Input: dimensioned drawing with shaded views. Units: mm. Origin: part minimum x, y, z. A direction names the side the tool comes from. Round coordinates to 2 decimals unless told otherwise and drop trailing zeros. Write each loop counter-clockwise with the first axis right and the second up, starting at its lowest first coordinate (ties: lowest second). Pieces come first, ordered by that corner, then holes. Notation, with made-up numbers: M 60,19.25 L 70,19.25 A26 ccw 70,42.25 Z; hole C -22.75,30 d5. An arc over 180 degrees is marked long. Answer in a Markdown table with one row per item. Add a question column.
Item 1: Cut plane C-C on x = 8.75. Return loops of the section in (y, z).
Item 2: Set-up query: the marked faces 1, 2, 3 and 4. Return all of +Z, -Z, +X, -X, +Y, -Y with unobstructed straight access to the full face (end or side cutting, diameter ignored); none if empty.
Item 3: Cut plane A-A on y = 10. Return loops of the section in (x, z).
Item 4: Contact query for flat-ended pins moving along their axis: pin 1 (3 mm diameter, centred on x = 9, y = 5.5, fed in from +Z); pin 2 (3 mm diameter, centred on x = 9.5, z = 5, fed in from +Y); pin 3 (2 mm diameter, centred on y = 13, z = 8, fed in from +X); pin 4 (3 mm diameter, centred on y = 14, z = 9.5, fed in from -X). Output: stop coordinate, or through.
Item 5: Cut plane B-B on z = 5. Return loops of the section in (x, y).
Item 6: Cut plane D-D on z = 8.5. Return loops of the section in (x, y), and give its area (3 significant figures).
Item 7: Mould query, pull axis Y, two halves, no side actions, for the marked faces 5, 6 and 7. Classes: released by +Y, released by -Y, zero draft, split by the parting line, or undercut.
Item 8: Material intervals for probe 1 along X at (y, z) = (10, 22.35); probe 2 along Z at (x, y) = (9.5, 13.4); probe 3 along X at (y, z) = (10, 18.6), sorted ascending.
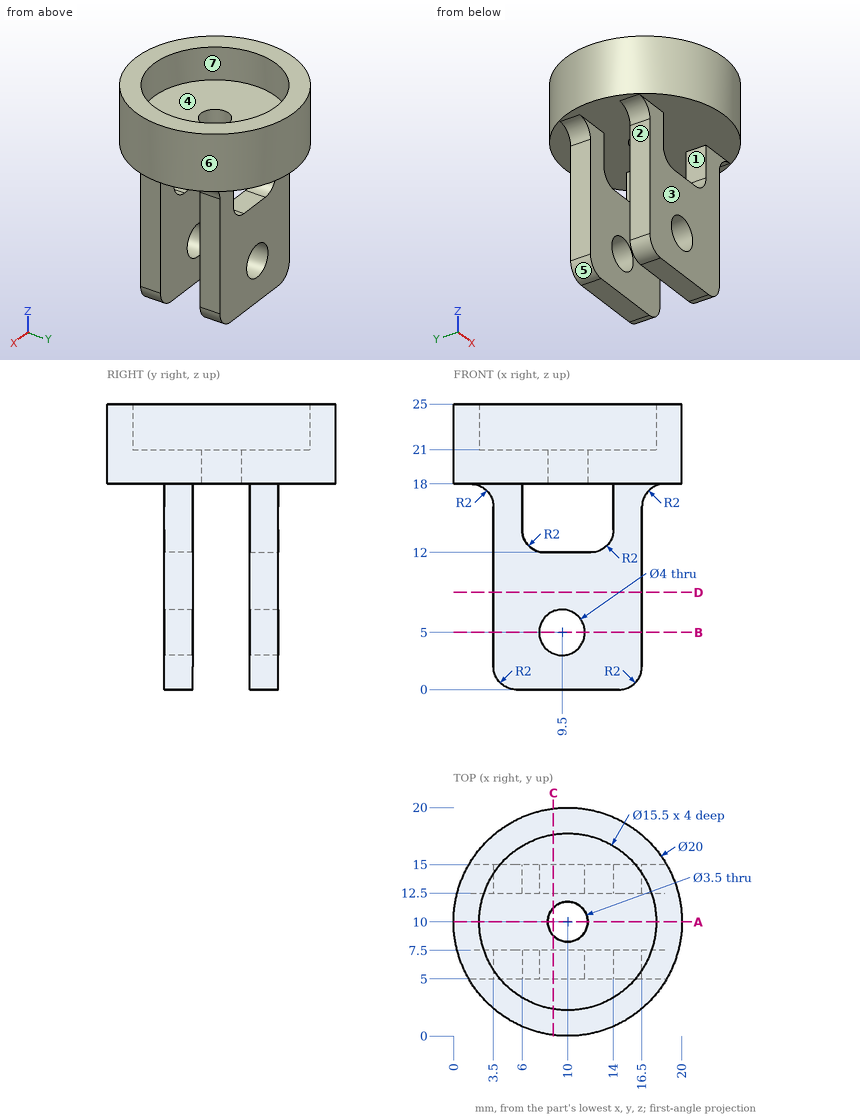
Results below:
| question | item | result |
|---|---|---|
| 1 | outline | M 0.08,18 L 8.78,18 L 8.78,21 L 2.35,21 L 2.35,25 L 0.08,25 Z; M 5,0 L 7.5,0 L 7.5,3.15 L 5,3.15 Z; M 5,6.85 L 7.5,6.85 L 7.5,12 L 5,12 Z; M 11.22,18 L 19.92,18 L 19.92,25 L 17.65,25 L 17.65,21 L 11.22,21 Z; M 12.5,0 L 15,0 L 15,3.15 L 12.5,3.15 Z; M 12.5,6.85 L 15,6.85 L 15,12 L 12.5,12 Z |
| 2 | face 1 | +Y, -Y |
| 2 | face 2 | -Z, -X, +Y, -Y |
| 2 | face 3 | -Z, +X, -X, -Y |
| 2 | face 4 | +Z |
| 3 | outline | M 0,18 L 8.25,18 L 8.25,21 L 2.25,21 L 2.25,25 L 0,25 Z; M 11.75,18 L 20,18 L 20,25 L 17.75,25 L 17.75,21 L 11.75,21 Z |
| 4 | pin 1 | z = 21 |
| 4 | pin 2 | through |
| 4 | pin 3 | x = 16.5 |
| 4 | pin 4 | x = 3.5 |
| 5 | outline | M 3.5,5 L 7.5,5 L 7.5,7.5 L 3.5,7.5 Z; M 3.5,12.5 L 7.5,12.5 L 7.5,15 L 3.5,15 Z; M 11.5,5 L 16.5,5 L 16.5,7.5 L 11.5,7.5 Z; M 11.5,12.5 L 16.5,12.5 L 16.5,15 L 11.5,15 Z |
| 6 | outline | M 3.5,5 L 16.5,5 L 16.5,7.5 L 3.5,7.5 Z; M 3.5,12.5 L 16.5,12.5 L 16.5,15 L 3.5,15 Z |
| 6 | area | 65.0 mm2 |
| 7 | face 5 | zero draft |
| 7 | face 6 | split by the parting line |
| 7 | face 7 | undercut |
| 8 | probe 1 | 0 to 2.25, 17.75 to 20 |
| 8 | probe 2 | 0 to 3, 7 to 12, 18 to 21 |
| 8 | probe 3 | 0 to 8.25, 11.75 to 20 |
